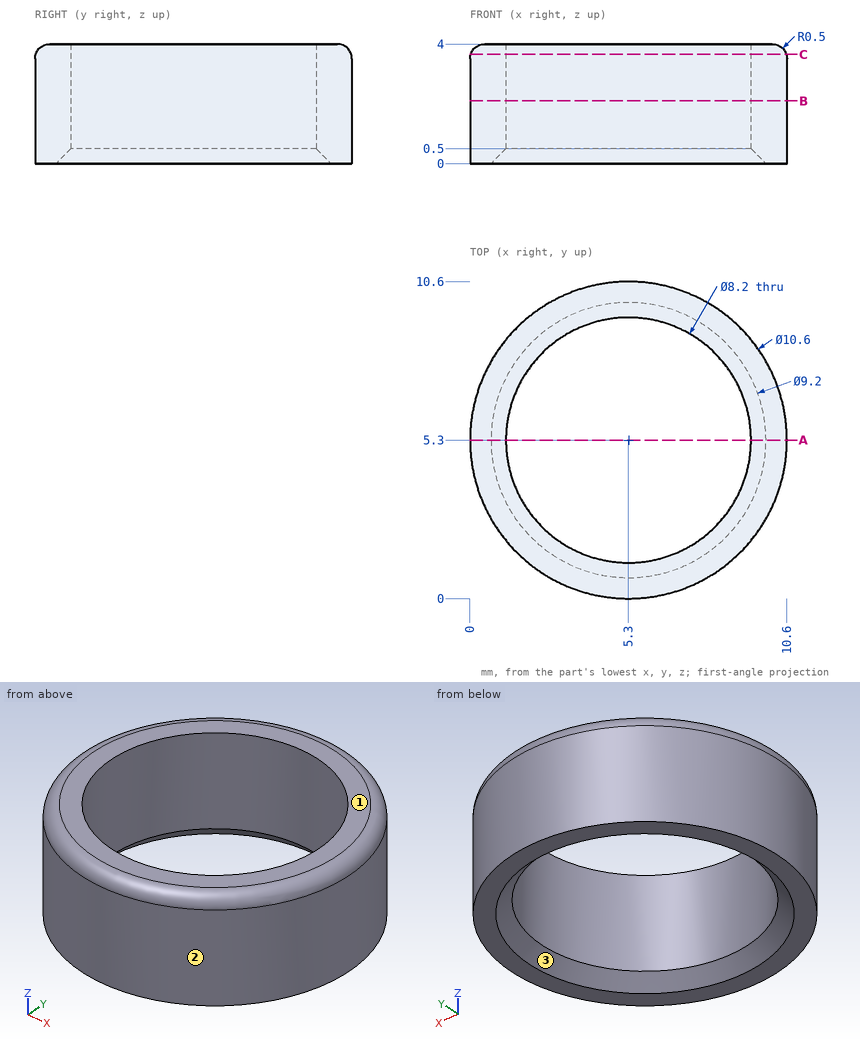
Could you check a few things on this drawing? It's one solid part, dimensions in mm from its lowest x, y, z. Coordinates: 2 decimals unless noted, no trailing zeros. Order: outer loops, then holes, each group sorted by start corner. A loop starts at its lowest first (then second) coordinate and runs counter-clockwise, first axis right, second up. Notation, with made-up numbers: (-26.75, 86.25) - (4.25, 86.25) arc R10 ccw to (4.25, 98.25) - close; hole circle Ø4 at (85, 81). An arc over 180 degrees is marked (long way). One line per question, with ' | ' between items.
(1) If I drill on L1, parallel to Y at x = 5.3, z = 2.1; L2, parallel to Y at x = 7.5, z = 1.8, over which ranges is the centre line in solid material (lowest first)?
Report:
L1: y = 0 to 1.2, 9.4 to 10.6 | L2: y = 0.48 to 1.84, 8.76 to 10.12
(2) Suppose I cut it at A-A on y = 5.3. List the corners of the cut face in (x, z) for me.
Report:
outline: (0, 0) - (0.7, 0) - (1.2, 0.5) - (1.2, 4) - (0.5, 4) arc R0.5 ccw to (0, 3.5) - close; (9.4, 0.5) - (9.9, 0) - (10.6, 0) - (10.6, 3.5) arc R0.5 ccw to (10.1, 4) - (9.4, 4) - close
(3) If we mould it in two halves opening along Y, with no side actions, what happens to the marked faces 1, 2 and 3? For each: pulls with the +Y half, pulls with the -Y half, needs draft (parallel to the pull), parting line crosses it, or undercut.
Report:
face 1: needs draft | face 2: parting line crosses it | face 3: undercut
(4) Will this pin go through, and if not, where does the flat tip stop? pin 1 (5 mm diameter, centred on x = 3, y = 7, fed in from -Z).
Report:
pin 1: stops at z = 0
(5) Suppose I cut it at B-B on z = 2.1. List the corners of the cut face in (x, y) for me, and give its area (3 significant figures).
Report:
outline: circle Ø10.6 at (5.3, 5.3); hole circle Ø8.2 at (5.3, 5.3) | area: 35.4 mm2
(6) Suppose I cut it at C-C on z = 3.65. List the corners of the cut face in (x, y) for me, and give its area (3 significant figures).
Report:
outline: circle Ø10.55 at (5.3, 5.3); hole circle Ø8.2 at (5.3, 5.3) | area: 34.7 mm2
